from build123d import *

# Parameters (mm, degrees)
SKETCH1_W                                     = 28.575
SKETCH1_H                                     = 137.16
BASE_FLANGE1_DEPTH                            = 1.5875
EDGE_FLANGE1_STRIP_W                          = 7.8232
EDGE_FLANGE1_STRIP_H                          = 1.5875
EDGE_FLANGE1_STRIP_CUT_DEPTH                  = 137.16
EDGE_FLANGE1_DEPTH                            = 137.16
CSK_FOR_8_FLAT_HEAD_MACHINE_SCREW1_AT_2_COUNT = 2
CSK_FOR_8_FLAT_HEAD_MACHINE_SCREW1_AT_2_PITCH = 27.432
CSK_FOR_8_FLAT_HEAD_MACHINE_SCREW1_AT_3_COUNT = 2
CSK_FOR_8_FLAT_HEAD_MACHINE_SCREW1_AT_3_PITCH = 54.864
CSK_FOR_8_FLAT_HEAD_MACHINE_SCREW1_AT_4_COUNT = 2
CSK_FOR_8_FLAT_HEAD_MACHINE_SCREW1_AT_4_PITCH = 82.296


# Sheet-metal steps are written as plain solids
with BuildPart() as part:
    # Sketch1 → Base-Flange1 (new body)
    with BuildSketch(Plane(origin=(0, 0, 0), x_dir=(1, 0, 0), z_dir=(0, 1, 0))):
        Rectangle(SKETCH1_W, SKETCH1_H)
    extrude(amount=-BASE_FLANGE1_DEPTH)

    # Edge-Flange1 strip (across the edge) → Edge-Flange1 strip cut (cut)
    with BuildSketch(Plane(origin=(-14.2875, 0, -68.58), x_dir=(1, 0, 0), z_dir=(0, 0, 1))):
        with Locations((-1.5875, -0.79375)):
            Rectangle(EDGE_FLANGE1_STRIP_W, EDGE_FLANGE1_STRIP_H)
    edge_flange1_strip_cut = extrude(amount=EDGE_FLANGE1_STRIP_CUT_DEPTH, mode=Mode.SUBTRACT)

    # Edge-Flange1 section (across the edge) → Edge-Flange1 (add)
    with BuildSketch(Plane(origin=(-14.2875, 0, -68.58), x_dir=(1, 0, 0), z_dir=(0, 0, 1))):
        with BuildLine():
            Line((0, 0.7366), (0, 4.7625))
            Line((0, 4.7625), (1.5875, 4.7625))
            Line((1.5875, 4.7625), (1.5875, 0.7366))
            ThreePointArc((1.5875, 0.7366), (1.803245145, 0.215745145), (2.3241, 0))
            Line((2.3241, 0), (2.3241, -1.5875))
            ThreePointArc((2.3241, -1.5875), (0.68071313, -0.90678687), (0, 0.7366))
        make_face()
    edge_flange1 = extrude(amount=EDGE_FLANGE1_DEPTH)

    # Mirror1: Edge-Flange1 strip cut, Edge-Flange1 across plane
    add(edge_flange1_strip_cut.mirror(Plane(origin=(0, 0, 0), x_dir=(0, 0, 1), z_dir=(1, 0, 0))), mode=Mode.SUBTRACT)
    add(edge_flange1.mirror(Plane(origin=(0, 0, 0), x_dir=(0, 0, 1), z_dir=(1, 0, 0))))

    # Sketch11 → CSK for #8 Flat Head Machine Screw1 (revolve, cut)
    with BuildSketch(Plane(origin=(0, 0, 41.148), x_dir=(0, 0, 1), z_dir=(1, 0, 0))):
        Polygon((0, 0), (0, 1.5875), (2.2479, 1.5875), (2.2479, 2.26450021), (4.2164, 0), align=None)
    csk_for_8_flat_head_machine_screw1 = revolve(axis=Axis((0, 6.35, 41.148), (0, -1, 0)), mode=Mode.SUBTRACT)

    # CSK for #8 Flat Head Machine Screw1 at 2: CSK for #8 Flat Head Machine Screw1 ×2
    with Locations(*[(0, 0, -i * CSK_FOR_8_FLAT_HEAD_MACHINE_SCREW1_AT_2_PITCH) for i in range(1, CSK_FOR_8_FLAT_HEAD_MACHINE_SCREW1_AT_2_COUNT)]):
        add(csk_for_8_flat_head_machine_screw1, mode=Mode.SUBTRACT)

    # CSK for #8 Flat Head Machine Screw1 at 3: CSK for #8 Flat Head Machine Screw1 ×2
    with Locations(*[(0, 0, -i * CSK_FOR_8_FLAT_HEAD_MACHINE_SCREW1_AT_3_PITCH) for i in range(1, CSK_FOR_8_FLAT_HEAD_MACHINE_SCREW1_AT_3_COUNT)]):
        add(csk_for_8_flat_head_machine_screw1, mode=Mode.SUBTRACT)

    # CSK for #8 Flat Head Machine Screw1 at 4: CSK for #8 Flat Head Machine Screw1 ×2
    with Locations(*[(0, 0, -i * CSK_FOR_8_FLAT_HEAD_MACHINE_SCREW1_AT_4_PITCH) for i in range(1, CSK_FOR_8_FLAT_HEAD_MACHINE_SCREW1_AT_4_COUNT)]):
        add(csk_for_8_flat_head_machine_screw1, mode=Mode.SUBTRACT)


solid = part.part
Source: CAD feature listing. Evaluate the final solid. Frame: model axes, mm. A direction names the side the tool comes from. Give positions to 0.01 mm unless a question says otherwise; leave off trailing zeros. Write each loop counter-clockwise with the first axis right and the second up, starting at its lowest first coordinate (ties: lowest second). Pieces come first, ordered by that corner, then holes. Notation, with made-up numbers: M 46,-9 L 82,-9 A20 cw 82,15 Z; hole C 3,8.5 d6. An arc over 180 degrees is marked long. Answer as a JSON object with one key per item and string values.
Q1. Cut plane B-B, the plane x = 0. Return the cut outline in (y, z), then the cut area to 3 significant figures.
Geometry check:
{"outline": "M -1.59,-68.58 L 0,-68.58 L 0,-45.36 L -1.59,-43.98 Z; M -1.59,-38.31 L 0,-36.93 L 0,-17.93 L -1.59,-16.55 Z; M -1.59,-10.88 L 0,-9.5 L 0,9.5 L -1.59,10.88 Z; M -1.59,16.55 L 0,17.93 L 0,36.93 L -1.59,38.31 Z; M -1.59,43.98 L 0,45.36 L 0,68.58 L -1.59,68.58 Z", "area": "173 mm^2"}
Q2. Cut plane A-A, the plane y = 3. Return the cut outline in (x, z), then the cut area to 3 significant figures.
Geometry check:
{"outline": "M -14.29,-68.58 L -12.7,-68.58 L -12.7,68.58 L -14.29,68.58 Z; M 12.7,-68.58 L 14.29,-68.58 L 14.29,68.58 L 12.7,68.58 Z", "area": "435 mm^2"}
Q3. Mould query, pull axis X, two halves, no side actions, for faces 3 (the face through (-1, -1, -68.58)), 4 (the face through (13.589, -0.925, -0.96)), 5 (the face through (-12.7, 3, -1)). Classes: +X half, -X half, draft (parallel to the pull), parting line (faces both ways), or undercut.
Geometry check:
{"face 3": "draft", "face 4": "+X half", "face 5": "undercut"}
Q4. Cut plane C-C, the plane z = -28. Return the cut outline in (x, y).
Geometry check:
{"outline": "M -14.29,0.74 A2.32 ccw -11.96,-1.59 L 11.96,-1.59 A2.32 ccw 14.29,0.74 L 14.29,4.76 L 12.7,4.76 L 12.7,0.74 A0.74 cw 11.96,0 L -11.96,0 A0.74 cw -12.7,0.74 L -12.7,4.76 L -14.29,4.76 Z"}
Q5. Access query for faces 1 (the face through (0, -1.588, -1)), 2 (the face through (0, 0, -1)). Directions: +Z, -Z, +X, -X, +Y, -Y. A direction counts if a zero-diameter tool reaches every point of the face in a straight line with its end or side. Return the directions, or none.
Geometry check:
{"face 1": "+Z, -Z, +X, -X, -Y", "face 2": "+Z, -Z, +Y"}
Q6. Ray query, line 1 along X through (y, z) = (3.5, 52); line 2 along Y through (x, z) = (9.5, 60.5); line 3 along Y through (x, z) = (-1.5, -45). Return the intervals inside material, ascending.
Geometry check:
{"line 1": "x = -14.29 to -12.7, 12.7 to 14.29", "line 2": "y = -1.59 to 0", "line 3": "y = -1.59 to -0.1"}
Q7. Cut plane D-D, the plane x = 7.5. Return the cut outline in (y, z), then the cut area to 3 significant figures.
Geometry check:
{"outline": "M -1.59,-68.58 L 0,-68.58 L 0,68.58 L -1.59,68.58 Z", "area": "218 mm^2"}
Q8. Contact query for a flat-ended pin moving along its axis: P1, Ø12, axis at x = -5.5, z = -50, coming from the +Y side. Output: stop coordinate, or through.
Geometry check:
{"P1": "stops at y = 0"}
